Can you work these out from the model? Positions are in its coordinate system, mm. Face numbers are marked on the shaded views. Round coordinates to 2 decimals unless told otherwise and drop trailing zeros. Order: outer loops, then holes, each group sorted by start corner. A loop starts at its lowest first (then second) coordinate and runs counter-clockwise, first axis right, second up. Notation, with made-up numbers: M -5,60.25 L 50,60.25 A23 ccw 50,85.25 Z; hole C -24,50 d11. An arc over 180 degrees is marked long. Answer as a JSON object with one key per item and string values. Group by question number.
from build123d import *

# Parameters (mm, degrees)
SKETCH2_R           = 1.6
BOSS_EXTRUDE1_DEPTH = 4


with BuildPart() as part:
    # Sketch1 → Revolve2 (revolve)
    with BuildSketch(Plane.XY):
        with BuildLine():
            ThreePointArc((6.530888148, 7.9), (3.470410639, 9.644622854), (0, 10.25))
            Line((0, 10.25), (0, 11.9))
            Line((0, 11.9), (12.5, 11.9))
            Line((12.5, 11.9), (12.5, 7.9))
            Line((12.5, 7.9), (6.530888148, 7.9))
        make_face()
    revolve(axis=Axis((0, 12.495, 0), (0, -1, 0)))

    # Sketch2 → Boss-Extrude1 (add)
    with BuildSketch(Plane(origin=(0, 11.9, 0), x_dir=(1, 0, 0), z_dir=(0, 1, 0))):
        with BuildLine():
            Line((-5.357142857, 11.293848786), (-19.642857143, 4.517539515))
            ThreePointArc((-19.642857143, 4.517539515), (-22.5, 0), (-19.642857143, -4.517539515))
            Line((-19.642857143, -4.517539515), (-5.357142857, -11.293848786))
            ThreePointArc((-5.357142857, -11.293848786), (-12.5, 0), (-5.357142857, 11.293848786))
        make_face()
        with Locations((-17.5, 0)):
            Circle(SKETCH2_R, mode=Mode.SUBTRACT)
        with BuildLine():
            Line((5.357142857, -11.293848786), (19.642857143, -4.517539515))
            ThreePointArc((19.642857143, -4.517539515), (22.5, 0), (19.642857143, 4.517539515))
            Line((19.642857143, 4.517539515), (5.357142857, 11.293848786))
            ThreePointArc((5.357142857, 11.293848786), (12.5, 0), (5.357142857, -11.293848786))
        make_face()
        with Locations((17.5, 0)):
            Circle(SKETCH2_R, mode=Mode.SUBTRACT)
    extrude(amount=-BOSS_EXTRUDE1_DEPTH)


solid = part.part
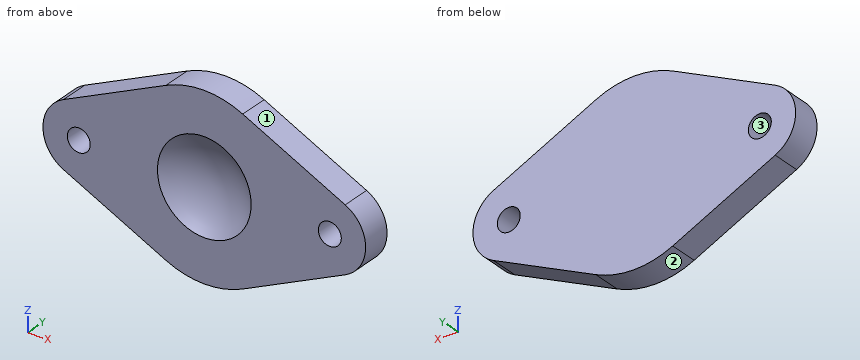
Item 1: Suppose I cut it at A-A, the plane y = 11.15. Write out the boundary of the cut face in (x, z).
Item 2: Suppose I cut it at C-C, the plane x = 16.5. Write out the boundary of the cut face in (y, z).
Item 3: Suppose I cut it at D-D, the plane z = -6. Write out the boundary of the cut face in (x, y), and give its area (3 significant figures).
Item 4: If we mould it in two halves opening along X, with no side actions, what happens to the marked faces 1, 2 and 3? For each: +X half, -X half, draft (parallel to the pull), parting line (faces both ways), or undercut.
Item 5: I'm going to push flat-ended pins straight in: pin 1 Ø1.5 at (x, y) = (-1, 10.5) entering from -Z; pin 2 Ø1 at (y, z) = (10.5, -10) entering from +X; pin 3 Ø1.5 at (x, y) = (-1.5, 11.5) entering from +Z; pin 4 Ø1.9 at (x, z) = (-17.5, 0) entering from +Y. Where does each tip first touch, or does it pass through?
Item 6: I need wall thicknesses on line 1 (X direction, y = 8.8, z = -0.75); line 2 (Z direction, x = -17.5, y = 10.6); line 3 (Z direction, x = 3, y = 8.2). Which ranges of each line are inside material? Lowest first, please.
Item 7: Suppose I cut it at B-B, the plane z = 0. Write out the boundary of the cut face in (x, y).
Computed:
{
 "1": {"outline": "M -19.64,-4.52 L -5.36,-11.29 A12.5 ccw 5.36,-11.29 L 19.64,-4.52 A5 ccw 19.64,4.52 L 5.36,11.29 A12.5 ccw -5.36,11.29 L -19.64,4.52 A5 ccw Z; hole C -17.5,0 d3.2; hole C 17.5,0 d3.2"},
 "2": {"outline": "M 7.9,-6.01 L 11.9,-6.01 L 11.9,-1.25 L 7.9,-1.25 Z; M 7.9,1.25 L 11.9,1.25 L 11.9,6.01 L 7.9,6.01 Z"},
 "3": {"outline": "M -16.52,7.9 L -2.58,7.9 A8.31 cw 2.58,7.9 L 16.52,7.9 L 16.52,11.9 L -16.52,11.9 Z", "area": "131 mm^2"},
 "4": {"face 1": "+X half", "face 2": "parting line", "face 3": "undercut"},
 "5": {"pin 1": "stops at z = -12.5", "pin 2": "stops at x = 9.14", "pin 3": "stops at z = 12.48", "pin 4": "passes through"},
 "6": {"line 1": "x = -22.44 to -18.91, -16.09 to -5.2, 5.2 to 16.09, 18.91 to 22.44", "line 2": "z = -5.53 to -1.6, 1.6 to 5.53", "line 3": "z = -12.13 to -5.37, 5.37 to 12.13"},
 "7": {"outline": "M -22.5,7.9 L -19.1,7.9 L -19.1,11.9 L -22.5,11.9 Z; M -15.9,7.9 L -6.53,7.9 A10.25 cw 6.53,7.9 L 15.9,7.9 L 15.9,11.9 L -15.9,11.9 Z; M 19.1,7.9 L 22.5,7.9 L 22.5,11.9 L 19.1,11.9 Z"}
}
